Input: part model. Units: mm. Frame: model coordinates. A direction names the side the tool comes from. Round coordinates to 2 decimals unless told otherwise and drop trailing zeros. Loops run counter-clockwise (first coordinate to the right, second up) from the corner with the lowest first, then second, coordinate; pieces in that order, holes last. Notation, with made-up numbers: (72.5, -17) -> (101.5, -17) arc R23 cw to (101.5, 9) -> close; hole circle Ø5 at (33, 13). An arc over 180 degrees is marked (long way). Answer in a Markdown table with one row per item. Add a question column.
Q1. Ray query, L1, parallel to X at y = 125, z = 1.7 (3 decimals); L2, parallel to X at y = 100.94, z = 3.65 (3 decimals); L3, parallel to X at y = -104.5, z = 3. Return the intervals inside material, ascending. Write a range as from..to.
Q2. Section D-D, the plane x = 73.5. Output: boundary loops of the cut face in (y, z), and give its area (3 significant figures).
Q3. Reachability of faces 5 (the face through (-175.69, -60.697, 2.465)), 6 (the face through (-3, 3, 5)) from +Z, -Z, +X, -X, +Y, -Y: full face, straight path, thin tool, end or side. Return the list, or none.
Q4. Mould query, pull axis Y, two halves, no side actions, for faces 1 (the face through (-112.987, -128.741, 2.465)), 2 (the face through (167.99, -33.48, 2.46)), 3 (the face through (190.764, -60.075, 2.465)), 4 (the face through (-3, 3, 0)). Classes: pulls with the +Y half, pulls with the -Y half, needs draft (parallel to the pull), parting line crosses it, or undercut.
Q5. Section C-C, the plane z = 3.9. Give the number of separate pieces and of enclosed holes in the cut face, and give its area (3 significant figures).
Q6. Section B-B, the plane x = 0. Output: boundary loops of the cut face in (y, z), and give its area (3 significant figures).
Q7. Section A-A, the plane y = 0. Output: boundary loops of the cut face in (x, z).
Q8. Pin query (flat end, axial travel): pin 1 (3 mm diameter, centred on x = -85, y = -65, fed in from -Z); pin 2 (1.5 mm diameter, centred on x = 10.5, z = 3.5, fed in from +Y); pin 3 (3 mm diameter, centred on x = 79.94, y = -63.41, fed in from -Z); pin 4 (1.5 mm diameter, centred on y = 185.5, z = 1.5, fed in from +X). Return the tip coordinate at first contact, or that it passes through.
Autodesk Inventor part; units mm, degrees
ref_plane "YZ Plane" through (0, 0, 0) normal (1, 0, 0) x (0, 1, 0)
ref_plane "XZ Plane" through (0, 0, 0) normal (0, 1, 0) x (-1, 0, 0)
ref_plane "XY Plane" through (0, 0, 0) normal (0, 0, 1) x (1, 0, 0)
sketch "Sketch1" plane through (0, 0, 0) normal (0, 0, 1) x (1, 0, 0)
  circle A0 centre (0, 0) radius 200
  line L0 (90.6699, 167.0448) -> (88.1699, 162.7147)
  line L1 (96.8301, 157.7147) -> (99.3301, 162.0448)
  line L2 (162.0448, 99.3301) -> (157.7147, 96.8301)
  line L3 (162.7147, 88.1699) -> (167.0448, 90.6699)
  line L4 (185, 5) -> (190, 5)
  line L5 (190, -5) -> (185, -5)
  line L6 (88.1699, -162.7147) -> (96.8301, -157.7147)
  line L7 (99.3301, -162.0448) -> (90.6699, -167.0448)
  line L8 (-5, -190) -> (-5, -185)
  line L9 (5, -185) -> (5, -190)
  line L10 (-99.3301, -162.0448) -> (-90.6699, -167.0448)
  line L11 (-88.1699, -162.7147) -> (-96.8301, -157.7147)
  line L12 (-190, 5) -> (-190, -5)
  line L13 (-190, -5) -> (-185, -5)
  line L14 (-185, -5) -> (-185, 5)
  line L15 (-167.0448, 90.6699) -> (-162.0448, 99.3301)
  line L16 (-157.7147, 96.8301) -> (-162.7147, 88.1699)
  line L17 (-99.3301, 162.0448) -> (-90.6699, 167.0448)
  line L18 (-88.1699, 162.7147) -> (-96.8301, 157.7147)
  line L19 (-190, -5) -> (-190, 5)
  line L20 (-185, 5) -> (-185, -5)
  line L21 (88.1699, 162.7147) -> (96.8301, 157.7147)
  line L22 (99.3301, 162.0448) -> (90.6699, 167.0448)
  line L23 (162.7147, 88.1699) -> (157.7147, 96.8301)
  line L24 (162.0448, 99.3301) -> (167.0448, 90.6699)
  line L25 (185, 5) -> (185, -5)
  line L26 (190, 5) -> (190, -5)
  line L27 (96.8301, -157.7147) -> (99.3301, -162.0448)
  line L28 (88.1699, -162.7147) -> (90.6699, -167.0448)
  line L29 (-5, -185) -> (5, -185)
  line L30 (-5, -190) -> (5, -190)
  line L31 (-99.3301, -162.0448) -> (-96.8301, -157.7147)
  line L32 (-90.6699, -167.0448) -> (-88.1699, -162.7147)
  line L33 (-190, 5) -> (-185, 5)
  line L34 (-162.0448, 99.3301) -> (-157.7147, 96.8301)
  line L35 (-167.0448, 90.6699) -> (-162.7147, 88.1699)
  line L36 (-99.3301, 162.0448) -> (-96.8301, 157.7147)
  line L37 (-90.6699, 167.0448) -> (-88.1699, 162.7147)
  line L38 (0, 142.5) -> (55, 142.5)
  line L39 (55, 142.5) -> (55, 182.5)
  line L40 (55, 182.5) -> (15, 182.5)
  line L41 (15, 182.5) -> (15, 187.5)
  line L42 (15, 187.5) -> (0, 187.5)
  line L43 (0, 142.5) -> (-55, 142.5)
  line L44 (-55, 142.5) -> (-55, 182.5)
  line L45 (-55, 182.5) -> (-15, 182.5)
  line L46 (-15, 182.5) -> (-15, 187.5)
  line L47 (-15, 187.5) -> (0, 187.5)
  line L48 (-123.4086, -71.25) -> (-95.9086, -118.8814)
  line L49 (-150.5496, -104.2404) -> (-154.8798, -106.7404)
  line L50 (-154.8798, -106.7404) -> (-162.3798, -93.75)
  line L51 (-95.9086, -118.8814) -> (-130.5496, -138.8814)
  line L52 (-130.5496, -138.8814) -> (-150.5496, -104.2404)
  line L53 (-123.4086, -71.25) -> (-150.9086, -23.6186)
  line L54 (-165.5496, -78.2596) -> (-169.8798, -80.7596)
  line L55 (-150.9086, -23.6186) -> (-185.5496, -43.6186)
  line L56 (-185.5496, -43.6186) -> (-165.5496, -78.2596)
  line L57 (-169.8798, -80.7596) -> (-162.3798, -93.75)
  line L58 (123.4086, -71.25) -> (150.9086, -23.6186)
  line L59 (165.5496, -78.2596) -> (169.8798, -80.7596)
  line L60 (169.8798, -80.7596) -> (162.3798, -93.75)
  line L61 (150.9086, -23.6186) -> (185.5496, -43.6186)
  line L62 (185.5496, -43.6186) -> (165.5496, -78.2596)
  line L63 (123.4086, -71.25) -> (95.9086, -118.8814)
  line L64 (150.5496, -104.2404) -> (154.8798, -106.7404)
  line L65 (95.9086, -118.8814) -> (130.5496, -138.8814)
  line L66 (130.5496, -138.8814) -> (150.5496, -104.2404)
  line L67 (154.8798, -106.7404) -> (162.3798, -93.75)
  line L68 (157.7147, 96.8301) -> (162.0448, 99.3301)
  line L69 (167.0448, 90.6699) -> (162.7147, 88.1699)
  line L70 (-99.3301, -162.0448) -> (-96.8301, -157.7147)
  line L71 (-88.1699, -162.7147) -> (-90.6699, -167.0448)
  line L72 (-99.3301, -162.0448) -> (-96.8301, -157.7147)
  line L73 (-88.1699, -162.7147) -> (-90.6699, -167.0448)
  line L74 (-99.3301, -162.0448) -> (-90.6699, -167.0448)
  circle A1 centre (14.945, 125) radius 1.73
  circle A2 centre (14.945, 100.94) radius 1.73
  circle A3 centre (-14.945, 125) radius 1.73
  circle A4 centre (-14.945, 100.94) radius 1.73
  circle A5 centre (-100.7807, -75.4427) radius 1.73
  circle A6 centre (-115.7257, -49.5573) radius 1.73
  circle A7 centre (-79.9441, -63.4127) radius 1.73
  circle A8 centre (-94.8891, -37.5273) radius 1.73
  circle A9 centre (115.7257, -49.5573) radius 1.73
  circle A10 centre (100.7807, -75.4427) radius 1.73
  circle A11 centre (94.8891, -37.5273) radius 1.73
  circle A12 centre (79.9441, -63.4127) radius 1.73
  dimension "d15" = 45
  dimension "d17" = 40
  dimension "d18" = 40
  dimension "d21" = 360
  dimension "d27" = 3.46
  dimension "d48" = 360
extrude "Extrusion1" add sketch "Sketch1" along normal blind 5 contours A0 | A1 | A2 | A3 | A4 | A5 | A6 | A7 | A8 | A9 | A10 | A11 | A12
extrude "Extrusion5" cut sketch "Sketch1" along normal blind 5 contours A1 | A2 | A3 | A4 | A5 | A6 | A7 | A8 | A9 | A10 | A11 | A12
properties part number "debanhxe"
Answer block:
| question | item | result |
|---|---|---|
| 1 | L1 | -156.125..-16.675, -13.215..13.215, 16.675..156.125 |
| 1 | L2 | -172.659..-16.675, -13.215..13.215, 16.675..172.659 |
| 1 | L3 | -170.53..-156.17, -151..-150.4, -104.21..104.21, 150.4..151, 156.17..170.53 |
| 2 | outline | (-186, 0) -> (186, 0) -> (186, 5) -> (-186, 5) -> close |
| 2 | area | 1,860 mm^2 |
| 3 | face 5 | +Z, -Z |
| 3 | face 6 | +Z, +X, -X, +Y, -Y |
| 4 | face 1 | undercut |
| 4 | face 2 | undercut |
| 4 | face 3 | parting line crosses it |
| 4 | face 4 | needs draft |
| 5 | separate pieces | 1 |
| 5 | enclosed holes | 24 |
| 5 | area | 111,000 mm^2 |
| 6 | outline | (-200, 0) -> (-190, 0) -> (-190, 5) -> (-200, 5) -> close; (-185, 0) -> (142.5, 0) -> (142.5, 5) -> (-185, 5) -> close; (187.5, 0) -> (200, 0) -> (200, 5) -> (187.5, 5) -> close |
| 6 | area | 1,750 mm^2 |
| 7 | outline | (-200, 0) -> (-190, 0) -> (-190, 5) -> (-200, 5) -> close; (-185, 0) -> (185, 0) -> (185, 5) -> (-185, 5) -> close; (190, 0) -> (200, 0) -> (200, 5) -> (190, 5) -> close |
| 8 | pin 1 | z = 0 |
| 8 | pin 2 | y = 199.76 |
| 8 | pin 3 | through |
| 8 | pin 4 | x = 76.6 |
